Source: CAD feature listing. Evaluate the final solid. Frame: model axes, mm. A direction names the side the tool comes from. Coordinates: 2 decimals unless noted, no trailing zeros. Write item = value, one per line.
from build123d import *

# Parameters (mm, degrees)
F_10_0MM_START                             = 12.85
F_10_0MM_CLEARANCE_DOWEL_HOLE1_OUTLINE_R   = 5.2
F_10_0MM_CLEARANCE_DOWEL_HOLE1_DEPTH       = 3.4
F_10_0MM_CLEARANCE_DOWEL_HOLE1_2_OUTLINE_R = 5.2
F_10_0MM_CLEARANCE_DOWEL_HOLE1_2_DEPTH     = 3.4
F_10_0MM_START_2                           = -16.25
F_10_0MM_CLEARANCE_DOWEL_HOLE1_3_OUTLINE_R = 5.2
F_10_0MM_CLEARANCE_DOWEL_HOLE1_3_DEPTH     = 3.4
F_10_0MM_CLEARANCE_DOWEL_HOLE1_4_OUTLINE_R = 5.2
F_10_0MM_CLEARANCE_DOWEL_HOLE1_4_DEPTH     = 3.4


# Read off the part's stored shape, not the designer's step: Ø10.0mm Clearance Dowel Hole1
with BuildPart() as part:
    # Sketch2 → Revolve1 (revolve)
    with BuildSketch(Plane(origin=(0, 0, 0), x_dir=(1, 0, 0), z_dir=(0, 1, 0))):
        with BuildLine():
            Line((0, 19.335223808), (0, 20.835223808))
            Line((0, 20.835223808), (3.5, 20.835223808))
            Line((3.5, 20.835223808), (3.5, 19.335223808))
            Line((3.5, 19.335223808), (15, 19.335223808))
            Line((15, 19.335223808), (15, 18.335223808))
            Line((15, 18.335223808), (7.652702684, 14.335223808))
            ThreePointArc((7.652702684, 14.335223808), (13.394084623, 9.201141077), (16.126453423, 2))
            Line((16.126453423, 2), (12.592160259, 2))
            ThreePointArc((12.592160259, 2), (10.383050167, 7.399646561), (6, 11.25))
            Line((6, 11.25), (6, 12.25))
            ThreePointArc((6, 12.25), (3.082974877, 13.314034437), (0, 13.683453923))
            Line((0, 13.683453923), (0, 14.335223808))
            Line((0, 14.335223808), (0, 19.335223808))
        make_face()
    revolve(axis=Axis((0, 0, 0), (0, 0, -1)))

    # Ø10.0mm Clearance Dowel Hole1 outline → Ø10.0mm Clearance Dowel Hole1 (cut)
    with BuildSketch(Plane(origin=(0, 0, 0), x_dir=(0.6183381372049325, 0.009621176242523823, 0.7858532821370949), z_dir=(0.7859121758046087, -0.0075697264639421865, -0.6182918009834247)).offset(F_10_0MM_START)):
        Circle(F_10_0MM_CLEARANCE_DOWEL_HOLE1_OUTLINE_R)
    extrude(amount=F_10_0MM_CLEARANCE_DOWEL_HOLE1_DEPTH, mode=Mode.SUBTRACT)

    # 10.0mm Clearance Dowel Hole1 2 outline → 10.0mm Clearance Dowel Hole1 2 (cut)
    with BuildSketch(Plane(origin=(0, 0, 0), x_dir=(0.9955100285365741, -0.07532499424889044, 0.05732301740587202), z_dir=(0.094656130721202, 0.792202117315513, -0.602873139422971)).offset(F_10_0MM_START)):
        Circle(F_10_0MM_CLEARANCE_DOWEL_HOLE1_2_OUTLINE_R)
    extrude(amount=F_10_0MM_CLEARANCE_DOWEL_HOLE1_2_DEPTH, mode=Mode.SUBTRACT)

    # 10.0mm Clearance Dowel Hole1 3 outline → 10.0mm Clearance Dowel Hole1 3 (cut)
    with BuildSketch(Plane(origin=(0, 0, 0), x_dir=(0.6223977246894614, -0.0005766674334576965, -0.7827009261244378), z_dir=(0.7827011385588891, 0.00045856135989200104, 0.6223975557632742)).offset(F_10_0MM_START_2)):
        Circle(F_10_0MM_CLEARANCE_DOWEL_HOLE1_3_OUTLINE_R)
    extrude(amount=F_10_0MM_CLEARANCE_DOWEL_HOLE1_3_DEPTH, mode=Mode.SUBTRACT)

    # 10.0mm Clearance Dowel Hole1 4 outline → 10.0mm Clearance Dowel Hole1 4 (cut)
    with BuildSketch(Plane(origin=(0, 0, 0), x_dir=(0.9995880641663693, -0.02335534361896009, -0.0166802248357377), z_dir=(0.02870020864262942, 0.8134339024051715, 0.5809488655998595)).offset(F_10_0MM_START_2)):
        Circle(F_10_0MM_CLEARANCE_DOWEL_HOLE1_4_OUTLINE_R)
    extrude(amount=F_10_0MM_CLEARANCE_DOWEL_HOLE1_4_DEPTH, mode=Mode.SUBTRACT)


solid = part.part
1) Material intervals for probe 1 along X at (y, z) = (1, -5.75); probe 2 along X at (y, z) = (0, -11.5); probe 3 along Z at (x, y) = (-11, 0), sorted ascending. Write a range as [from, to].
Answer block:
probe_1 = [-11.85, -11.34], [11.34, 11.84]
probe_2 = [-7.27, -6], [6, 7.3]
probe_3 = [-19.34, -16.16], [-6.81, -6.45]
2) First-contact query: pin 1 Ø10 at (x, z) = (10.5, -7.5) entering from -Y; pin 2 Ø4 at (x, z) = (3.5, -7.5) entering from -Y; pin 3 Ø3 at (x, y) = (-10.5, -2) entering from -Z. Flat tips, straight axial feed; report the tip coordinate or a pass-through.
Answer block:
pin_1 = -14.2
pin_2 = -14.99
pin_3 = -19.34
3) Pull-direction query (Y, two-part tool) for faces 1 (the cylindrical face through (-1.08, -8.49, -12.4)), 2 (the cylindrical face through (3.233, 1.341, -20.075)), 3 (the flat face through (0, -4, -19.335)); classes: +Y half, -Y half, draft (parallel to the pull), parting line (faces both ways), or undercut.
Answer block:
face_1 = undercut
face_2 = parting line
face_3 = draft
4) Reachability of faces 4 (the cylindrical face through (-14.985, -0.66, -18.828)), 5 (the flat face through (0, 0, -20.835)), 6 (the flat face through (-10, 8, -2)), 7 (the flat face through (1.14, 9.44, -8.73)), 8 (the cylindrical face through (-6, 0, -12)) from +Z, -Z, +X, -X, +Y, -Y: full face, straight path, thin tool, end or side. Return the list, or none.
Answer block:
face_4 = -Z
face_5 = -Z, +X, -X, +Y, -Y
face_6 = +Z, +X, -X, +Y, -Y
face_7 = none
face_8 = +Z
